Geometry: see drawing. Coordinates: mm, zero at the bounding-box minimum. A direction names the side the tool comes from. Give positions to 0.01 mm unless a question says otherwise; leave off trailing zeros. Write each loop counter-clockwise with the first axis right and the second up, starting at its lowest first coordinate (ties: lowest second). Pieces come first, ordered by that corner, then holes. Notation, with made-up numbers: (-30, -31.5) -> (-26, -31.5) arc R15 ccw to (-26, -9.5) -> close; hole circle Ø4 at (-12, 5). An arc over 180 degrees is marked (long way). Answer as a JSON object with one key per item and string values. Group by question number.
Item 1: Pull-direction query (Y, two-part tool) for the marked faces 4, 5 and 6; classes: pulls with the +Y half, pulls with the -Y half, needs draft (parallel to the pull), parting line crosses it, or undercut.
Item 2: Section query B-B on z = 5.5. Return the cut outline in (x, y), plus the area to 3 significant figures.
Item 3: Section query A-A on y = 7.25. Return the cut outline in (x, z), plus the area to 3 significant figures.
Item 4: Access query for the marked faces 1, 2 and 3. Directions: +Z, -Z, +X, -X, +Y, -Y. A direction counts if a zero-diameter tool reaches every point of the face in a straight line with its end or side. Return the directions, or none.
Item 5: Section query D-D on z = 9. Return the cut outline in (x, y), plus the area to 3 significant figures.
Item 6: Ray query, probe 1 along X at (y, z) = (12.25, 9); probe 2 along Z at (x, y) = (1.5, 5); probe 3 along X at (y, z) = (13.75, 4.25). Return the intervals inside material, ascending. Write a range as from..to.
Item 7: Section query C-C on x = 4. Return the cut outline in (y, z), plus the area to 3 significant figures.
Item 8: First-contact query: pin 1 Ø3 at (x, y) = (4, 7.25) entering from +Z; pin 2 Ø2.5 at (y, z) = (12.5, 6.5) entering from +X; pin 3 Ø1 at (y, z) = (10, 10) entering from -X; pin 4 Ø0.9 at (y, z) = (1.5, 8) entering from -X. Flat tips, straight axial feed; report the tip coordinate or a pass-through.
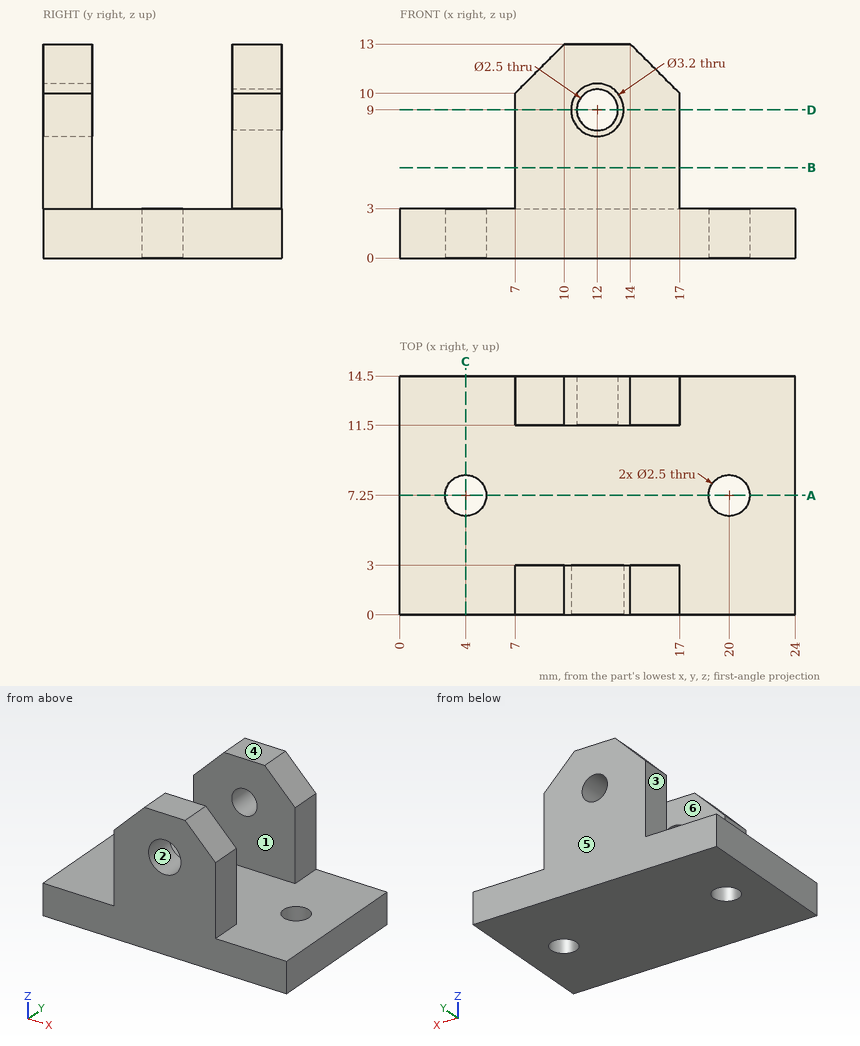
Worked answers:
{
 "1": {"face 4": "needs draft", "face 5": "pulls with the +Y half", "face 6": "undercut"},
 "2": {"outline": "(7, 0) -> (17, 0) -> (17, 3) -> (7, 3) -> close; (7, 11.5) -> (17, 11.5) -> (17, 14.5) -> (7, 14.5) -> close", "area": "60.0 mm^2"},
 "3": {"outline": "(0, 0) -> (2.75, 0) -> (2.75, 3) -> (0, 3) -> close; (5.25, 0) -> (18.75, 0) -> (18.75, 3) -> (5.25, 3) -> close; (21.25, 0) -> (24, 0) -> (24, 3) -> (21.25, 3) -> close", "area": "57.0 mm^2"},
 "4": {"face 1": "+Z, +X, -X", "face 2": "-Y", "face 3": "+Z, -X, +Y, -Y"},
 "5": {"outline": "(7, 0) -> (10.4, 0) -> (10.4, 3) -> (7, 3) -> close; (7, 11.5) -> (10.75, 11.5) -> (10.75, 14.5) -> (7, 14.5) -> close; (13.25, 11.5) -> (17, 11.5) -> (17, 14.5) -> (13.25, 14.5) -> close; (13.6, 0) -> (17, 0) -> (17, 3) -> (13.6, 3) -> close", "area": "42.9 mm^2"},
 "6": {"probe 1": "7..10.75, 13.25..17", "probe 2": "0..3", "probe 3": "7..17"},
 "7": {"outline": "(0, 0) -> (6, 0) -> (6, 3) -> (0, 3) -> close; (8.5, 0) -> (14.5, 0) -> (14.5, 3) -> (8.5, 3) -> close", "area": "36.0 mm^2"},
 "8": {"pin 1": "z = 3", "pin 2": "x = 17", "pin 3": "through", "pin 4": "x = 7"}
}
